```python
from build123d import *

# Parameters (mm, degrees)
BOSS_EXTRUDE1_DEPTH = 10
FILLET1_R           = 2
FILLET2_R           = 2
BLOCK_START         = 73.5
BLOCK_OUTLINE_R     = 1.65
BLOCK_DEPTH         = 4
BLOCK_START_2       = 77.5
BLOCK_2_DEPTH       = 0.2
CUT_EXTRUDE1_START  = -0.2
CUT_EXTRUDE1_DEPTH  = 0.2
FILLET4_R           = 4


# Read off the part's stored shape, not the designer's step: block
with BuildPart() as part:
    # Sketch1 → Boss-Extrude1 (new body)
    with BuildSketch(Plane(origin=(0, 0, 0), x_dir=(1, 0, 0), z_dir=(0, 1, 0))):
        with BuildLine():
            Line((24, -55), (24, 0))
            Line((24, 0), (29, 0))
            Line((29, 0), (29, -55))
            Line((29, -55), (30.5, -56.5))
            Line((30.5, -56.5), (30.5, -70.5))
            Line((30.5, -70.5), (30.5, -77.5))
            Line((30.5, -77.5), (-30.5, -77.5))
            Line((-30.5, -77.5), (-30.5, -70.5))
            Line((-30.5, -70.5), (-30.5, -56.5))
            Line((-30.5, -56.5), (-29, -55))
            Line((-29, -55), (-29, 0))
            Line((-29, 0), (-24, 0))
            Line((-24, 0), (-24, -55))
            Line((-24, -55), (-22.5, -56.5))
            Line((-22.5, -56.5), (-22.5, -70.5))
            ThreePointArc((-22.5, -70.5), (-21.914213562, -71.914213562), (-20.5, -72.5))
            Line((-20.5, -72.5), (20.5, -72.5))
            ThreePointArc((20.5, -72.5), (21.914213562, -71.914213562), (22.5, -70.5))
            Line((22.5, -70.5), (22.5, -56.5))
            Line((22.5, -56.5), (24, -55))
        make_face()
        with BuildLine():
            Line((24.5, -58.5), (24.5, -70.5))
            ThreePointArc((24.5, -70.5), (26.5, -72.5), (28.5, -70.5))
            Line((28.5, -70.5), (28.5, -58.5))
            ThreePointArc((28.5, -58.5), (26.5, -56.5), (24.5, -58.5))
        make_face(mode=Mode.SUBTRACT)
        with BuildLine():
            Line((-28.5, -70.5), (-28.5, -58.5))
            ThreePointArc((-28.5, -58.5), (-26.5, -56.5), (-24.5, -58.5))
            Line((-24.5, -58.5), (-24.5, -70.5))
            ThreePointArc((-24.5, -70.5), (-26.5, -72.5), (-28.5, -70.5))
        make_face(mode=Mode.SUBTRACT)
    extrude(amount=BOSS_EXTRUDE1_DEPTH)

    # Fillet1
    fillet1_edges = [part.edges().sort_by_distance(p)[0] for p in [
        (30.5, 5, 77.5),
        (-30.5, 5, 77.5),
        (-30.5, 5, 56.5),
        (-29, 5, 55),
        (-24, 5, 55),
        (-22.5, 5, 56.5),
        (22.5, 5, 56.5),
        (24, 5, 55),
        (29, 5, 55),
        (30.5, 5, 56.5),
    ]]
    fillet(fillet1_edges, radius=FILLET1_R)

    # Fillet2
    fillet2_edges = [part.edges().sort_by_distance(p)[0] for p in [
        (-29, 5, 0),
        (-24, 5, 0),
        (24, 5, 0),
        (29, 5, 0),
    ]]
    fillet(fillet2_edges, radius=FILLET2_R)


with BuildPart() as body_2:
    # block outline → block (new body)
    with BuildSketch(Plane.XY.offset(BLOCK_START)):
        with BuildLine():
            Line((-10, 0), (-10, -2))
            ThreePointArc((-10, -2), (-8.535533906, -5.535533906), (-5, -7))
            Line((-5, -7), (5, -7))
            ThreePointArc((5, -7), (8.535533906, -5.535533906), (10, -2))
            Line((10, -2), (10, 0))
            Line((10, 0), (-10, 0))
        make_face()
        with Locations((-4.5, -4)):
            Circle(BLOCK_OUTLINE_R, mode=Mode.SUBTRACT)
        with Locations((4.5, -4)):
            Circle(BLOCK_OUTLINE_R, mode=Mode.SUBTRACT)
    extrude(amount=BLOCK_DEPTH)

    # block 2 outline → block 2 (add)
    with BuildSketch(Plane.XY.offset(BLOCK_START_2)):
        with BuildLine():
            ThreePointArc((-3, -0.5), (-3.2, -0.7), (-3, -0.9))
            Line((-3, -0.9), (3, -0.9))
            ThreePointArc((3, -0.9), (3.2, -0.7), (3, -0.5))
            Line((3, -0.5), (-3, -0.5))
        make_face()
    extrude(amount=BLOCK_2_DEPTH)


with BuildPart() as part_1:
    add(part.part)

    # Combine1: union body 2
    add(body_2.part)

    # Sketch3 → Cut-Extrude1 (cut)
    with BuildSketch(Plane.XY.offset(77.7).offset(CUT_EXTRUDE1_START)):
        with BuildLine():
            Line((-3, -0.9), (3, -0.9))
            ThreePointArc((3, -0.9), (3.2, -0.7), (3, -0.5))
            Line((3, -0.5), (-3, -0.5))
            ThreePointArc((-3, -0.5), (-3.2, -0.7), (-3, -0.9))
        make_face()
    extrude(amount=CUT_EXTRUDE1_DEPTH, mode=Mode.SUBTRACT)

    # Fillet4
    # the kernel refuses this fillet: 4 mm, written as the material it adds along each edge
    with BuildSketch(Plane(origin=(10, 0, 73.5), x_dir=(1, 0, 0), z_dir=(0, 0, 1))) as fillet4_piece_1:
        with BuildLine():
            CenterArc((3.774964387, -4), FILLET4_R, 90, 77.160411594)
            Line((-0.125019785, -3.111111111), (-0.515018202, -3.022222222))
            ThreePointArc((-0.515018202, -3.022222222), (-0.4, -2), (-0.4, 0))
            Line((-0.4, 0), (0, 0.4))
            Line((0, 0.4), (3.774964387, 0.4))
            Line((3.774964387, 0.4), (3.774964387, 0))
        make_face()
    extrude(amount=4)
    with BuildSketch(Plane(origin=(-10, 0, 73.5), x_dir=(-1, 0, 0), z_dir=(0, 0, 1))) as fillet4_piece_2:
        with BuildLine():
            CenterArc((3.774964387, 4), FILLET4_R, 192.839588406, 77.160411594)
            Line((-0.125019785, 3.111111111), (-0.515018202, 3.022222222))
            ThreePointArc((-0.515018202, 3.022222222), (-0.4, 2), (-0.4, 0))
            Line((-0.4, 0), (0, -0.4))
            Line((0, -0.4), (3.774964387, -0.4))
            Line((3.774964387, -0.4), (3.774964387, 0))
        make_face()
    extrude(amount=4)


solid = part_1.part
```
Work out the finished part from the listing and answer in its coordinate system (mm). A direction names the side the tool comes from. Give positions to 0.01 mm unless a question says otherwise; leave off trailing zeros. Write each loop counter-clockwise with the first axis right and the second up, starting at its lowest first coordinate (ties: lowest second). Pieces come first, ordered by that corner, then holes. Notation, with made-up numbers: (67.25, -27.75) -> (118.25, -27.75) arc R21 ccw to (118.25, 9.25) -> close; hole circle Ø8 at (47, -11). An arc over 180 degrees is marked (long way). Write item = value, one per line.
Q1. Section C-C on y = 6.75 is taken. State how many separate pieces and enclosed holes the cut face has, and give its area (3 significant figures).
Computed values:
separate_pieces = 1
enclosed_holes = 2
area = 1,010 mm^2
Q2. Section D-D on x = -18 is taken. Determine the outline of the cut face in (y, z).
Computed values:
outline = (0, 72.5) -> (10, 72.5) -> (10, 77.5) -> (0, 77.5) -> close
Q3. A tool of negligible diameter and unlimited length cuts with its end or side. For faces 1 (the cylindrical face through (-26.5, 4.9, 72.5)), 2 (the flat face through (29, 5, 28)), 3 (the flat face through (-29, 5, 28)), 4 (the flat face through (22.5, 5, 64)), from which of +Z, -Z, +X, -X, +Y, -Y can it reach the whole face along a straight path? Write none if from no direction.
Computed values:
face_1 = +Y, -Y
face_2 = -Z, +X, +Y, -Y
face_3 = -Z, -X, +Y, -Y
face_4 = -Z, +Y, -Y
Q4. For a pull along X with two mould halves and no side action, classify faces 5 (the cylindrical face through (-11.25, -0.9, 75.47)), 6 (the flat face through (0, 3, 77.5)), 7 (the flat face through (24.5, 5, 64)) as pulls with the +X half, pulls with the -X half, needs draft (parallel to the pull), parting line crosses it, or undercut.
Computed values:
face_5 = pulls with the -X half
face_6 = needs draft
face_7 = undercut
Q5. Section A-A on z = 39.5 is taken. Determine the outline of the cut face in (x, y), and give its area (3 significant figures).
Computed values:
outline = (-29, 0) -> (-24, 0) -> (-24, 10) -> (-29, 10) -> close; (24, 0) -> (29, 0) -> (29, 10) -> (24, 10) -> close
area = 100 mm^2
Q6. Flat-ended cylindrical pins translate along their axes: pin 1 Ø6 at (y, z) = (-2, 48.5) entering from +X; pin 2 Ø2 at (x, y) = (-3.5, 2.5) entering from -Z; pin 3 Ø5 at (y, z) = (4.5, 34) entering from -X. Find the tip coordinate at first contact, or state that the pin passes through.
Computed values:
pin_1 = 29
pin_2 = 72.5
pin_3 = -29
Q7. Section B-B on y = -4 is taken. Determine the outline of the cut face in (x, z), and give its area (3 significant figures).
Computed values:
outline = (-9.58, 73.5) -> (-6.15, 73.5) -> (-6.15, 77.5) -> (-9.58, 77.5) -> close; (-2.85, 73.5) -> (2.85, 73.5) -> (2.85, 77.5) -> (-2.85, 77.5) -> close; (6.15, 73.5) -> (9.58, 73.5) -> (9.58, 77.5) -> (6.15, 77.5) -> close
area = 50.3 mm^2
Q8. Consider line 1 along Y through (x, z) = (4.5, 75.75); line 2 along X through (y, z) = (6, 21); line 3 along Z through (x, y) = (26, 9.25). Determine where each line is inside the solid, lowest interval first.
Computed values:
line_1 = -7 to -5.65, -2.35 to 10
line_2 = -29 to -24, 24 to 29
line_3 = 0 to 56.56, 72.44 to 77.5
